Could you check a few things on this model? Use its own coordinates, in mm. Coordinates: 2 decimals unless noted, no trailing zeros. Write each loop counter-clockwise with the first axis right and the second up, starting at its lowest first coordinate (ties: lowest second). Pieces come first, ordered by that corner, then holes.
```python
from build123d import *

# Parameters (mm, degrees)
SKETCH1_RX          = 40.067331288
SKETCH1_RY          = 16.556748466
BOSS_EXTRUDE1_DEPTH = 18.288
BOSS_EXTRUDE2_DEPTH = 24.13
SKETCH4_R           = 5.089278313
CUT_EXTRUDE1_DEPTH  = 49.784


with BuildPart() as part:
    # Sketch1 → Boss-Extrude1 (new body)
    with BuildSketch(Plane.XY):
        with Locations(Location((-74.44297323, -2.317944785), (0, 0, 180))):
            Ellipse(SKETCH1_RX, SKETCH1_RY)
    extrude(amount=BOSS_EXTRUDE1_DEPTH)

    # Sketch3 → Boss-Extrude2 (add)
    with BuildSketch(Plane(origin=(0, 0, 0), x_dir=(-1, 0, 0), z_dir=(0, 0, -1))):
        with BuildLine():
            Line((74.44297323, -18.874693252), (-48.961371747, -18.874693252))
            Line((-48.961371747, -18.874693252), (-48.961371747, 14.238803681))
            Line((-48.961371747, 14.238803681), (77.490698265, 14.190836373))
            add(Edge.make_bspline(
                [(74.44297323, -18.874693252), (113.013283161, -18.874693252), (114.48127378, -2.948096616), (115.949264398, 12.978500019), (77.490698265, 14.190836373)],
                knots=[4.71238898, 4.71238898, 4.71238898, 6.245115993, 6.245115993, 7.777843005, 7.777843005, 7.777843005], degree=2, weights=[1, 0.720437409, 1, 0.720437409, 1]))
        make_face()
    extrude(amount=-BOSS_EXTRUDE2_DEPTH)

    # Sketch4 → Cut-Extrude1 (cut)
    with BuildSketch(Plane(origin=(0, 0, 0), x_dir=(-1, 0, 0), z_dir=(0, 0, -1))):
        with Locations((114.510304518, -2.317944785)):
            Circle(SKETCH4_R)
    extrude(amount=-CUT_EXTRUDE1_DEPTH, mode=Mode.SUBTRACT)


solid = part.part
```
Item 1: I want a section at A-A, the plane y = -3. List the corners of the cut face in (x, z) for me.
Item 2: Will this pin go through, and if not, where does the flat tip stop? pin 1 Ø8 at (x, z) = (9.5, 13.5) entering from +Y.
Item 3: If I drill on line 1 along Y through (x, z) = (-33, 4); line 2 along X through (y, z) = (-2.5, 11.5); line 3 along Y through (x, z) = (-78.5, 22.75), over which ranges is the centre line in solid material (lowest first)?
Item 4: If we mould it in two halves opening along Y, with no side actions, what happens to faces 1 (the flat face through (-14, -18.875, 12)), 2 (the cylindrical face through (-109.42, -2.23, 11.9)), 3 (the flat face through (-33, -2, 0))? For each: released by +Y, released by -Y, zero draft, split by the parting line, or undercut.
Taken from the geometry:
1. outline: (-109.47, 0) - (48.96, 0) - (48.96, 24.13) - (-109.47, 24.13) - close
2. pin 1: stops at y = 14.23
3. line 1: y = -18.87 to 14.21
3. line 2: x = -109.42 to 48.96
3. line 3: y = -18.79 to 14.15
4. face 1: released by -Y
4. face 2: undercut
4. face 3: zero draft
